Design review of the part shown in the three views and the two pictorial views. Dimensions are in mm from the part's minimum x, y and z. Round coordinates to 2 decimals unless told otherwise and drop trailing zeros. Order: outer loops, then holes, each group sorted by start corner. A loop starts at its lowest first (then second) coordinate and runs counter-clockwise, first axis right, second up.
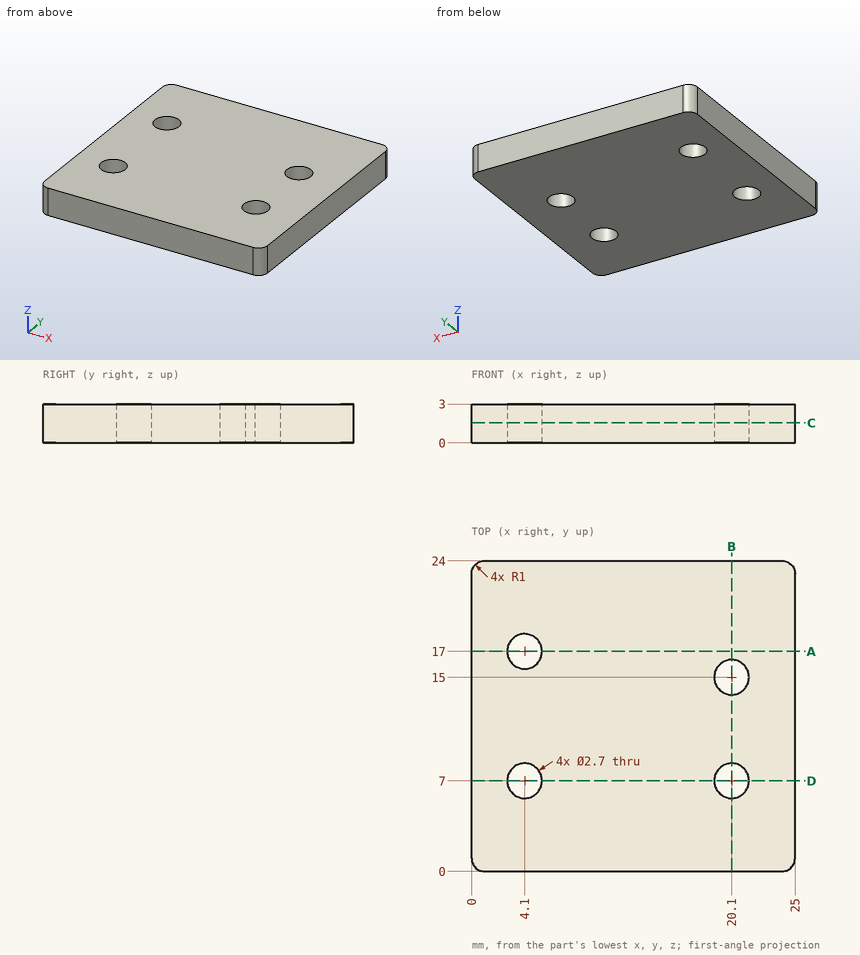
(1) Consider section A-A (y = 17). Write out the cut boundary in (x, z).
Data:
outline: (0, 0) - (2.75, 0) - (2.75, 3) - (0, 3) - close; (5.45, 0) - (25, 0) - (25, 3) - (5.45, 3) - close
(2) Consider section D-D (y = 7). Write out the cut boundary in (x, z), and give its area (3 significant figures).
Data:
outline: (0, 0) - (2.75, 0) - (2.75, 3) - (0, 3) - close; (5.45, 0) - (18.75, 0) - (18.75, 3) - (5.45, 3) - close; (21.45, 0) - (25, 0) - (25, 3) - (21.45, 3) - close
area: 58.8 mm2
(3) To check wall thickness, follow probe 1 along Y at (x, z) = (4.1, 0.9); probe 2 along Y at (x, z) = (20.1, 1.4); probe 3 along X at (y, z) = (7.75, 1.2). State the ranges of each line that lie inside material, in increasing order.
Data:
probe 1: y = 0 to 5.65, 8.35 to 15.65, 18.35 to 24
probe 2: y = 0 to 5.65, 8.35 to 13.65, 16.35 to 24
probe 3: x = 0 to 2.98, 5.22 to 18.98, 21.22 to 25
(4) Consider section B-B (x = 20.1). Write out the cut boundary in (y, z).
Data:
outline: (0, 0) - (5.65, 0) - (5.65, 3) - (0, 3) - close; (8.35, 0) - (13.65, 0) - (13.65, 3) - (8.35, 3) - close; (16.35, 0) - (24, 0) - (24, 3) - (16.35, 3) - close
(5) Insertion check: pin 1 (2.5 mm diameter, centred on x = 20.1, y = 7, fed in from +Z). The pin has a flat end and moves straight along its axis. Give the tip position at first contact, or say it passes through.
Data:
pin 1: passes through
(6) Consider section C-C (z = 1.55). Write out the cut boundary in (x, y), and give its area (3 significant figures).
Data:
outline: (0, 1) arc R1 ccw to (1, 0) - (24, 0) arc R1 ccw to (25, 1) - (25, 23) arc R1 ccw to (24, 24) - (1, 24) arc R1 ccw to (0, 23) - close; hole circle Ø2.7 at (4.1, 7); hole circle Ø2.7 at (4.1, 17); hole circle Ø2.7 at (20.1, 7); hole circle Ø2.7 at (20.1, 15)
area: 576 mm2
